```python
from build123d import *

# Parameters (mm, degrees)
PAD005_DEPTH = 67.5
FILLET_R     = 1
FILLET001_R  = 1


with BuildPart() as part:
    # Sketch005 → Pad005 (new body, symmetric)
    with BuildSketch(Plane.YZ):
        Polygon((0, 13.5), (0, -13.5), (-6.5, -13.5), (-6.5, -17.5), (-7.5, -17.5), (-7.5, -12.5), (-1, -12.5), (-1, 12.5), (-7.5, 12.5), (-7.5, 17.5), (-6.5, 17.5), (-6.5, 13.5), align=None)
    extrude(amount=PAD005_DEPTH, both=True)

    # Fillet
    fillet_edges = [part.edges().sort_by_distance(p)[0] for p in [
        (0, -7.5, -12.5),
    ]]
    fillet(fillet_edges, radius=FILLET_R)

    # Fillet001
    fillet001_edges = [part.edges().sort_by_distance(p)[0] for p in [
        (0, -7.5, 12.5),
    ]]
    fillet(fillet001_edges, radius=FILLET001_R)


solid = part.part
```
Part model, mm, in its own coordinate system. A direction names the side the tool comes from. Round coordinates to 2 decimals unless told otherwise and drop trailing zeros. Loops run counter-clockwise (first coordinate to the right, second up) from the corner with the lowest first, then second, coordinate; pieces in that order, holes last.
Item 1: 3-axis set-ups, long thin cutter, end or side, ignore diameter. For faces 1 (the face through (1, -3, -13.5)), 2 (the face through (1, -4, -12.5)), 3 (the face through (-67.5, -0.7, 0.1)), 4 (the face through (1, -7.5, 15)), 5 (the face through (1, -6.5, 16)): which of +Z, -Z, +X, -X, +Y, -Y reach the whole face in a straight line?
Item 2: Drill centre lines: line 1 (Z direction, x = 34, y = -3.75); line 2 (Z direction, x = -56.5, y = -0.5); line 3 (Y direction, x = 50, z = 10). Where is each one in solid material? Low to high.
Item 3: Cut at B-B, the plane x = 24.5. Give the cut face in (y, z), then the cut area to 3 significant figures.
Item 4: Cut at A-A, the plane y = -4. Give the cut face in (x, z), then the cut area to 3 significant figures.
Item 5: Cut at C-C, the plane z = 7. Give the cut face in (x, y).
Item 6: Drop flat-ended pins along their axis: P1, Ø1.5, axis at x = 39.5, y = -2, coming from the +Z side; P2, Ø1, axis at x = 45, z = -11, coming from the -Y side; P3, Ø3, axis at x = 3, y = -4, coming from the -Z side. Give the stop position or say it passes through.
Item 7: Mould opens along Z. For faces 6 (the face through (1, -7.5, -16)), 7 (the face through (1, -3, 13.5)), 8 (the face through (1, -1, 0)) say: +Z half, -Z half, draft (parallel to the pull), parting line (faces both ways), or undercut.
A:
1. face 1: -Z, +X, -X, +Y
1. face 2: +X, -X, -Y
1. face 3: +Z, -Z, -X, +Y, -Y
1. face 4: +Z, -Z, +X, -X, -Y
1. face 5: +Z, +X, -X, +Y
2. line 1: z = -13.5 to -12.5, 12.5 to 13.5
2. line 2: z = -13.5 to 13.5
2. line 3: y = -1 to 0
3. outline: (-7.5, -17.5) - (-6.5, -17.5) - (-6.5, -13.5) - (0, -13.5) - (0, 13.5) - (-6.5, 13.5) - (-6.5, 17.5) - (-7.5, 17.5) - (-7.5, 13.5) arc R1 ccw to (-6.5, 12.5) - (-1, 12.5) - (-1, -12.5) - (-6.5, -12.5) arc R1 ccw to (-7.5, -13.5) - close
3. area: 47.6 mm2
4. outline: (-67.5, -13.5) - (67.5, -13.5) - (67.5, -12.5) - (-67.5, -12.5) - close; (-67.5, 12.5) - (67.5, 12.5) - (67.5, 13.5) - (-67.5, 13.5) - close
4. area: 270 mm2
5. outline: (-67.5, -1) - (67.5, -1) - (67.5, 0) - (-67.5, 0) - close
6. P1: stops at z = 13.5
6. P2: stops at y = -1
6. P3: stops at z = -13.5
7. face 6: draft
7. face 7: +Z half
7. face 8: undercut
